```python
from build123d import *

# Parameters (mm, degrees)
F1_DEPTH  = 70
F3_DEPTH  = 80
F5_DEPTH  = 100
F8_DEPTH  = 70
F10_DEPTH = 80


with BuildPart() as f1:
    # F0 (on Right) → F1 (new body)
    with BuildSketch(Plane.YZ):
        Polygon((-8.8, 0), (0, 0), (-1.227845609, 10), (-10.027845609, 10), align=None)
    extrude(amount=F1_DEPTH)

    # F2 (on face) → F3 (join)
    with BuildSketch(Plane.YZ.offset(70)):
        Polygon((0, 0), (-1.227845609, 10), (-10.027845609, 10), (-8.8, 0), align=None)
        Polygon((-10.027845609, 10), (-1.227845609, 10), (-2.4556912181, 20), (-11.2556912181, 20), align=None)
    extrude(amount=F3_DEPTH)

    # F4 (on face) → F5 (join)
    with BuildSketch(Plane.YZ.offset(150)):
        Polygon((-8.8, 0), (0, 0), (-2.4556912181, 20), (-11.2556912181, 20), align=None)
        Polygon((-11.2556912181, 20), (-2.4556912181, 20), (-3.6835368271, 30), (-12.4835368271, 30), align=None)
    extrude(amount=F5_DEPTH)

    # F7 (on face) → F8 (join)
    with BuildSketch(Plane(origin=(0, 0, 0), x_dir=(0, -1, 0), z_dir=(-1, 0, 0))):
        Polygon((2.4556912181, 20), (1.227845609, 10), (6.4556912181, 10), (6.4556912181, 20), align=None)
    extrude(amount=-F8_DEPTH)

    # F9 (on face) → F10 (join)
    with BuildSketch(Plane(origin=(150, 0, 0), x_dir=(0, -1, 0), z_dir=(-1, 0, 0))):
        Polygon((2.4556912181, 20), (7.6835368271, 20), (7.6835368271, 30), (3.6835368271, 30), align=None)
    extrude(amount=F10_DEPTH)


solid = f1.part
```
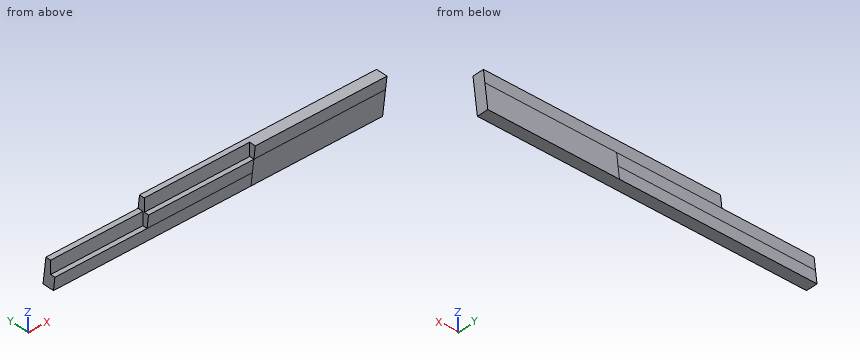
Read the model definition and answer for the solid it produces. Units are mm, in the model's axes. Round coordinates to 2 decimals unless told otherwise and drop trailing zeros. Write each loop counter-clockwise with the first axis right and the second up, starting at its lowest first coordinate (ties: lowest second). Pieces come first, ordered by that corner, then holes. Notation, with made-up numbers: (47, 71.5) - (71, 71.5) arc R17 cw to (71, 102.5) - close; hole circle Ø11 at (64.5, -39.5). An arc over 180 degrees is marked (long way). Use CSV: the item, a comma, the result in double quotes.
Q1. Straight lines are drawn through the part: line 1 along X through (y, z) = (-8.25, 28); line 2 along Y through (x, z) = (95.5, 19.75) (3 decimals); line 3 along Z through (x, y) = (15, -5.75). For each, find the intervals that lie inside material, in ascending order.
Values:
line 1,"x = 150 to 250"
line 2,"y = -11.225 to -2.425"
line 3,"z = 0 to 20"
Q2. Find section D-D, the plane z = 15.25. Write down the section's boundary in (x, y), then the cut area to 3 significant figures.
Values:
outline,"(0, -6.46) - (70, -6.46) - (70, -10.67) - (250, -10.67) - (250, -1.87) - (0, -1.87) - close"
area,"1,900 mm²"
Q3. Find section C-C, the plane x = 118. Write down the section's boundary in (y, z), then the cut area to 3 significant figures.
Values:
outline,"(-11.26, 20) - (-8.8, 0) - (0, 0) - (-3.68, 30) - (-7.68, 30) - (-7.68, 20) - close"
area,"222 mm²"
Q4. Each of these flat-tipped pins is pushed along its axis until it touches: pin 1 Ø3 at (x, y) = (92.5, -10) entering from +Z; pin 2 Ø8 at (x, z) = (46.5, 16.5) entering from -Y; pin 3 Ø11 at (x, z) = (128, 23) entering from -Y. Where does it stop, or does it pass through?
Values:
pin 1,"stops at z = 20"
pin 2,"stops at y = -6.46"
pin 3,"stops at y = -11.26"
Q5. Find section B-B, the plane z = 25.5. Write down the section's boundary in (x, y), then the cut area to 3 significant figures.
Values:
outline,"(70, -7.68) - (150, -7.68) - (150, -11.93) - (250, -11.93) - (250, -3.13) - (70, -3.13) - close"
area,"1,240 mm²"
Q6. Find section A-A, the plane x = 30.5. Write down the section's boundary in (y, z), then the cut area to 3 significant figures.
Values:
outline,"(-10.03, 10) - (-8.8, 0) - (0, 0) - (-2.46, 20) - (-6.46, 20) - (-6.46, 10) - close"
area,"134 mm²"
